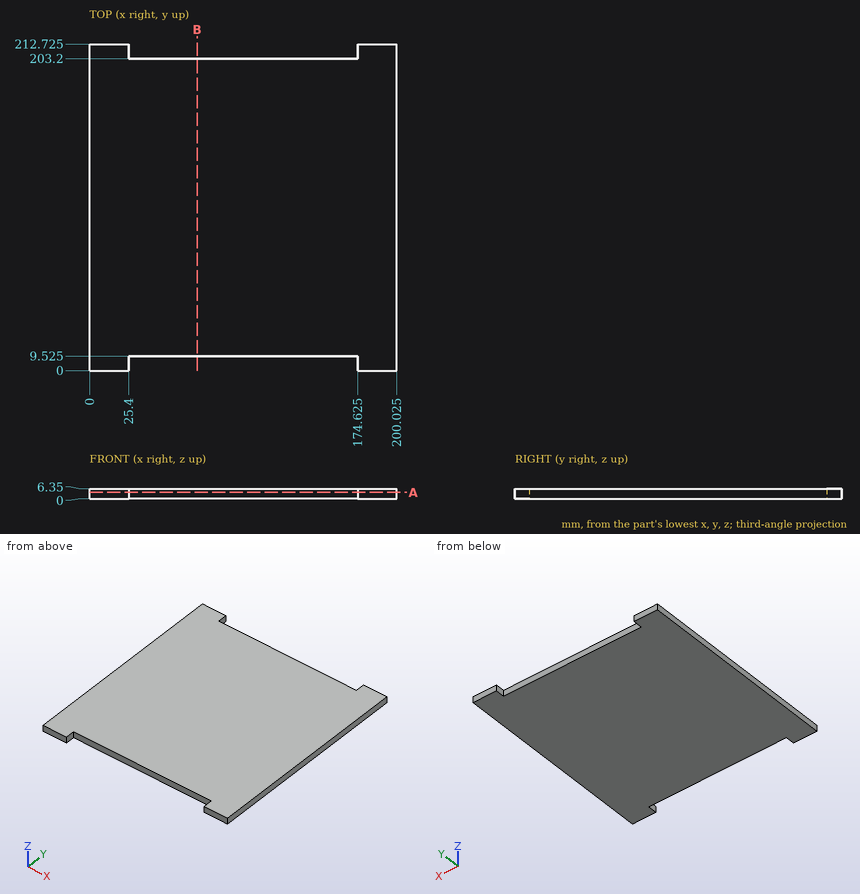
Job drawing, mm, ordinate dimensions from the low corner. One solid piece. Coordinates: 2 decimals unless noted, no trailing zeros. Order: outer loops, then holes, each group sorted by start corner. A loop starts at its lowest first (then second) coordinate and runs counter-clockwise, first axis right, second up. Notation, with made-up numbers: (-34, 3.5) - (12, 3.5) arc R5 ccw to (12, 11.5) - close; hole circle Ø2 at (-3.75, -26.75). An arc over 180 degrees is marked (long way). Write each question's results on one line, items separated by ' | '. Start each with the question number.
Item 1: Flat gauge pin, fed straight in: pin 1 (1 mm diameter, centred on x = 89, z = 0.5, fed in from +Y). Where does the tip first touch, or does it go through?
Item 2: Wall check: probe 1 along Y at (x, z) = (101, 2.5) (3 decimals). Give the ranges that are in metal, low to high. Write a range as [from, to].
Item 3: Band-saw the part on A-A on z = 4. Write the cut outline in (x, y) (3 decimals).
Item 4: Band-saw the part on B-B on x = 70. Write the cut outline in (y, z) (3 decimals), and give its area (3 significant figures).
Numbers:
1) pin 1: y = 203.2
2) probe 1: [9.525, 203.2]
3) outline: (0, 0) - (25.4, 0) - (25.4, 9.525) - (174.625, 9.525) - (174.625, 0) - (200.025, 0) - (200.025, 212.725) - (174.625, 212.725) - (174.625, 203.2) - (25.4, 203.2) - (25.4, 212.725) - (0, 212.725) - close
4) outline: (9.525, 0) - (203.2, 0) - (203.2, 6.35) - (9.525, 6.35) - close | area: 1,230 mm^2
